```python
from build123d import *

# Parameters (mm, degrees)
BOSS_EXTRUDE1_DEPTH     = 12.7
CUT_EXTRUDE1_REACH      = 105.136
CUT_EXTRUDE1_END_RADIUS = 66.15
SKETCH4_R               = 1.55
BOSS_EXTRUDE2_START     = -12.7
BOSS_EXTRUDE2_DEPTH     = 12.7
BOSS_EXTRUDE4_START     = -12.7
BOSS_EXTRUDE4_DEPTH     = 12.7
CUT_EXTRUDE2_REACH      = 88.037
CUT_EXTRUDE2_END_RADIUS = 44.45
SKETCH9_R               = 1.55
BOSS_EXTRUDE3_START     = -22.86
SKETCH9_3_R             = 2.54
SKETCH9_3_R_2           = 1.55
BOSS_EXTRUDE3_DEPTH     = 7.62
F_6_CLEARANCE_HOLE1_D   = 3.7973


with BuildPart() as part:
    # Sketch1 → Boss-Extrude1 (new body)
    with BuildSketch(Plane(origin=(0, 0, 0), x_dir=(1, 0, 0), z_dir=(0, 1, 0))):
        with BuildLine():
            ThreePointArc((-33.160552015, 64.471914738), (-45.240476214, 56.65288441), (-55.538222126, 46.602101702))
            Line((-55.538222126, 46.602101702), (-50.673839912, 42.520400381))
            ThreePointArc((-50.673839912, 42.520400381), (-43.444022026, 49.884260546), (-35.15688403, 56.034061117))
            ThreePointArc((-35.15688403, 56.034061117), (0, 38.783252378), (35.15688403, 56.034061117))
            ThreePointArc((35.15688403, 56.034061117), (43.444022026, 49.884260546), (50.673839912, 42.520400381))
            Line((50.673839912, 42.520400381), (55.538222126, 46.602101702))
            ThreePointArc((55.538222126, 46.602101702), (45.240476214, 56.65288441), (33.160552015, 64.471914738))
            ThreePointArc((33.160552015, 64.471914738), (0, 45.133252378), (-33.160552015, 64.471914738))
        make_face()
    extrude(amount=BOSS_EXTRUDE1_DEPTH)

    # Cut-Extrude1: up to this cylinder (the profile starts outside it)
    cut_extrude1_end = Plane(origin=(0, 6.35, 0), z_dir=(0, -1, 0)) * Cylinder(CUT_EXTRUDE1_END_RADIUS, 343.572, mode=Mode.PRIVATE)
    # Sketch4 → Cut-Extrude1 (cut, up to the surface)
    with BuildSketch(Plane(origin=(-45.240476214, 12.7, -56.65288441), x_dir=(-0.7814190953093677, 0, 0.6240065684637377), z_dir=(-0.6240065684637377, 0, -0.7814190953093677)), mode=Mode.PRIVATE) as cut_extrude1_sk1:
        with Locations((0, -6.35)):
            Circle(SKETCH4_R)
    cut_extrude1_tool1 = extrude(cut_extrude1_sk1.sketch, amount=-CUT_EXTRUDE1_REACH, mode=Mode.PRIVATE) - cut_extrude1_end
    cut_extrude1 = cut_extrude1_tool1.solids().sort_by_distance((-45.240476, 6.35, -56.652884))[0]
    add(cut_extrude1, mode=Mode.SUBTRACT)

    # Sketch5 → Boss-Extrude2 (add)
    with BuildSketch(Plane(origin=(0, 12.7, 0), x_dir=(1, 0, 0), z_dir=(0, 1, 0)).offset(BOSS_EXTRUDE2_START)):
        with BuildLine():
            Line((-48.180298109, 40.428070373), (-50.673839912, 42.520400381))
            ThreePointArc((-50.673839912, 42.520400381), (-48.57209115, 44.906285321), (-46.358122599, 47.188419862))
            Line((-46.358122599, 47.188419862), (-44.098596788, 45.292452587))
            ThreePointArc((-44.098596788, 45.292452587), (-43.707256341, 40.81941082), (-48.180298109, 40.428070373))
        make_face()
    boss_extrude2 = extrude(amount=BOSS_EXTRUDE2_DEPTH)

    # Sketch10 → Boss-Extrude4 (add)
    with BuildSketch(Plane(origin=(0, 12.7, 0), x_dir=(1, 0, 0), z_dir=(0, 1, 0)).offset(BOSS_EXTRUDE4_START)):
        with BuildLine():
            Line((-3.175, 38.896790239), (-3.175, 35.947188775))
            ThreePointArc((-3.175, 35.947188775), (0, 32.772188775), (3.175, 35.947188775))
            Line((3.175, 35.947188775), (3.175, 38.896790239))
            ThreePointArc((3.175, 38.896790239), (0, 38.783252378), (-3.175, 38.896790239))
        make_face()
    extrude(amount=BOSS_EXTRUDE4_DEPTH)

    # Cut-Extrude2: up to this cylinder (the profile starts inside it)
    cut_extrude2_end = Plane(origin=(0, 6.35, -83.233252378), z_dir=(0, -1, 0)) * Cylinder(CUT_EXTRUDE2_END_RADIUS, 265.974, mode=Mode.PRIVATE)
    # Sketch9 → Cut-Extrude2 (cut, up to the surface)
    with BuildSketch(Plane(origin=(0, 0, 0), x_dir=(0, 0, -1), z_dir=(1, 0, 0)), mode=Mode.PRIVATE) as cut_extrude2_sk1:
        with Locations((48.26, 6.35)):
            Circle(SKETCH9_R)
    cut_extrude2_tool1 = extrude(cut_extrude2_sk1.sketch, amount=-CUT_EXTRUDE2_REACH, mode=Mode.PRIVATE) & cut_extrude2_end
    cut_extrude2 = cut_extrude2_tool1.solids().sort_by_distance((0, 6.35, -48.26))[0]
    add(cut_extrude2, mode=Mode.SUBTRACT)

    # Sketch9<3> → Boss-Extrude3 (add)
    with BuildSketch(Plane(origin=(0, 0, 0), x_dir=(0, 0, -1), z_dir=(1, 0, 0)).offset(BOSS_EXTRUDE3_START)):
        with Locations((48.26, 6.35)):
            Circle(SKETCH9_3_R)
        with Locations((48.26, 6.35)):
            Circle(SKETCH9_3_R_2, mode=Mode.SUBTRACT)
    boss_extrude3 = extrude(amount=-BOSS_EXTRUDE3_DEPTH)

    # Mirror1: Cut-Extrude1, Boss-Extrude2, Cut-Extrude2, Boss-Extrude3 across plane
    add(cut_extrude1.mirror(Plane(origin=(0, 0, 0), x_dir=(0, 0, 1), z_dir=(1, 0, 0))), mode=Mode.SUBTRACT)
    add(boss_extrude2.mirror(Plane(origin=(0, 0, 0), x_dir=(0, 0, 1), z_dir=(1, 0, 0))))
    add(cut_extrude2.mirror(Plane(origin=(0, 0, 0), x_dir=(0, 0, 1), z_dir=(1, 0, 0))), mode=Mode.SUBTRACT)
    add(boss_extrude3.mirror(Plane(origin=(0, 0, 0), x_dir=(0, 0, 1), z_dir=(1, 0, 0))))

    # #6 Clearance Hole1 (through all)
    with Locations(Plane(origin=(0, 12.7, 0), x_dir=(1, 0, 0), z_dir=(0, 1, 0))):
        with Locations((-46.139447448, 42.86026148), (46.139447448, 42.86026148), (0, 35.947188775)):
            Hole(F_6_CLEARANCE_HOLE1_D / 2)


solid = part.part
```
Check sheet for the modelled part. Datum: model origin and axes. Units: mm. A direction names the side the tool comes from. Give positions to 0.01 mm unless a question says otherwise; leave off trailing zeros. Order: outer loops, then holes, each group sorted by start corner. A loop starts at its lowest first (then second) coordinate and runs counter-clockwise, first axis right, second up. Notation, with made-up numbers: M -29.5,-9 L 17.5,-9 A29 ccw 17.5,22 Z; hole C 45.25,-28 d4. An arc over 180 degrees is marked long. Answer in a Markdown table with one row per item.
1) Release check for a two-part mould opening along X. For faces 1 (the cylindrical face through (-0.07, 6.261, -32.773)), 2 (the cylindrical face through (45.398, 9.083, -56.527)), 3 (the cylindrical face through (0.563, 6.261, -45.137)) record: +X half, -X half, draft (parallel to the pull), parting line (faces both ways), or undercut.
Filled sheet:
| item | result |
|---|---|
| face 1 | parting line |
| face 2 | +X half |
| face 3 | undercut |
2) Thickness scan on L1, parallel to Y at x = -27.05, z = -48.26; L2, parallel to Z at x = 0, y = 5.5; L3, parallel to X at y = 2, z = -43.5. Record the ranges inside material, lowest first. Write a range as [from, to].
Filled sheet:
| item | result |
|---|---|
| L1 | y = [0, 4.8], [7.9, 12.7] |
| L2 | z = [-45.13, -37.85], [-34.05, -32.77] |
| L3 | x = [-51.84, -47.93], [-44.35, -43.03], [-19.93, 19.93], [43.03, 44.35], [47.93, 51.84] |
3) Cross-section at A-A, the plane x = 0. Enter the section's corners in (y, z), plus the area to 3 significant figures.
Filled sheet:
| item | result |
|---|---|
| outline | M 0,-45.13 L 12.7,-45.13 L 12.7,-37.85 L 0,-37.85 Z; M 0,-34.05 L 12.7,-34.05 L 12.7,-32.77 L 0,-32.77 Z |
| area | 109 mm2 |
4) Access from +Z, -Z, +X, -X, +Y, -Y to the whole of each face (thin tool, end or side, straight path). Record for faces 4 (the flat face through (3.175, 6, -37)), 5 (the flat face through (30.48, 5, -47)), 6 (the flat face through (-3.175, 6, -37)), 7 (the cylindrical face through (39.66, 6.26, -52.94)).
Filled sheet:
| item | result |
|---|---|
| face 4 | +Z, +X, +Y, -Y |
| face 5 | +Z, +Y, -Y |
| face 6 | +Z, -X, +Y, -Y |
| face 7 | +Y, -Y |
5) Cross-section at B-B, the plane z = -48.26. Count the separate pieces of the cut face and the enclosed holes in it, plus the area to 3 significant figures.
Filled sheet:
| item | result |
|---|---|
| separate pieces | 6 |
| enclosed holes | 0 |
| area | 474 mm2 |
6) Cross-section at D-D, the plane y = 11.5. Enter the section's corners in (x, z) (3 decimals).
Filled sheet:
| item | result |
|---|---|
| outline | M -55.538,-46.602 A72.5 ccw -33.161,-64.472 A38.1 cw 33.161,-64.472 A72.5 ccw 55.538,-46.602 L 48.18,-40.428 A3.175 ccw 44.099,-45.292 L 46.358,-47.188 A66.15 cw 35.157,-56.034 A44.45 ccw 3.175,-38.897 L 3.175,-35.947 A3.175 ccw -3.175,-35.947 L -3.175,-38.897 A44.45 ccw -35.157,-56.034 A66.15 cw -46.358,-47.188 L -44.099,-45.292 A3.175 ccw -48.18,-40.428 Z; hole C -46.139,-42.86 d3.797; hole C 0,-35.947 d3.797; hole C 46.139,-42.86 d3.797 |
7) Gauge pin test, flat ends, axial feed: P1, Ø3, axis at y = 6.35, z = -48.26, coming from the -X side; P2, Ø5.5, axis at y = 5.5, z = -47.5, coming from the -X side; P3, Ø1.5, axis at x = 30, z = -48.5, coming from the +Y side; P4, Ø3, axis at x = 46.14, z = -42.86, coming from the -Y side. Record the tip position at first contact, or that the pin passes through.
Filled sheet:
| item | result |
|---|---|
| P1 | stops at x = -55.41 |
| P2 | stops at x = -55.54 |
| P3 | stops at y = 8.89 |
| P4 | passes through |
